Can you work these out from the model? Positions are in its coordinate system, mm. Give positions to 0.01 mm unless a question says otherwise; leave off trailing zeros. Loops run counter-clockwise (first coordinate to the right, second up) from the corner with the lowest first, then second, coordinate; pieces in that order, holes last. Notation, with made-up numbers: (39.5, 11.5) - (50.5, 11.5) arc R19 ccw to (50.5, 36.5) - close; hole circle Ø8 at (73.5, -17.75). An arc over 180 degrees is marked (long way). Answer as a JSON object with one key per item and string values. Group by question number.
Item 1: Thinking about a two-plate mould opening in Y: for faces 1 (the cylindrical face through (6.466, -2.681, 9.86)), 2 (the cylindrical face through (-1.08, -4.88, 9.87)), 3 (the flat face through (6, 2, 0)), which applies, pulls with the +Y half, pulls with the -Y half, needs draft (parallel to the pull), parting line crosses it, or undercut?
Item 2: Please list where these lines run through material, in increasing order: L1, parallel to Y at x = 0, z = 5.5; L2, parallel to Y at x = -4.5, z = 2; L3, parallel to X at y = -3.25, z = 4.
Item 3: Suppose I cut it at A-A on x = 0. Write out the boundary of the cut face in (y, z).
Item 4: Suppose I cut it at B-B on z = 13.75. Write out the boundary of the cut face in (x, y).
Item 5: Will these pins go through, and if not, where does the flat tip stop? pin 1 (5 mm diameter, centred on y = 4, z = 16, fed in from +X); pin 2 (3 mm diameter, centred on x = -2.5, z = 10.5, fed in from -Y).
from build123d import *

# Parameters (mm, degrees)
SKETCH_R        = 7
SKETCH_R_2      = 5
PAD_DEPTH       = 20
CHAMFER_SIZE    = 1
CHAMFER001_SIZE = 1


with BuildPart() as part:
    # Sketch → Pad (new body)
    with BuildSketch(Plane.XY):
        Circle(SKETCH_R)
        Circle(SKETCH_R_2, mode=Mode.SUBTRACT)
    extrude(amount=PAD_DEPTH)

    # Chamfer
    chamfer_edges = [part.edges().sort_by_distance(p)[0] for p in [
        (-5, 0, 20),
    ]]
    chamfer(chamfer_edges, length=CHAMFER_SIZE)

    # Chamfer001
    chamfer001_edges = [part.edges().sort_by_distance(p)[0] for p in [
        (-5, 0, 0),
    ]]
    chamfer(chamfer001_edges, length=CHAMFER001_SIZE)


solid = part.part
Worked out:
{
 "1": {"face 1": "parting line crosses it", "face 2": "undercut", "face 3": "needs draft"},
 "2": {"L1": "y = -7 to -5, 5 to 7", "L2": "y = -5.36 to -2.18, 2.18 to 5.36", "L3": "x = -6.2 to -3.8, 3.8 to 6.2"},
 "3": {"outline": "(-7, 0) - (-6, 0) - (-5, 1) - (-5, 19) - (-6, 20) - (-7, 20) - close; (5, 1) - (6, 0) - (7, 0) - (7, 20) - (6, 20) - (5, 19) - close"},
 "4": {"outline": "circle Ø14 at (0, 0); hole circle Ø10 at (0, 0)"},
 "5": {"pin 1": "stops at x = 6.84", "pin 2": "stops at y = -6.93"}
}
